CAD build for the part. Positions are in the model's coordinates, mm. A direction names the side the tool comes from. Round coordinates to 2 decimals unless told otherwise and drop trailing zeros. Order: outer loops, then holes, each group sorted by start corner. A loop starts at its lowest first (then second) coordinate and runs counter-clockwise, first axis right, second up. Notation, with made-up numbers: (-17, 89) - (34, 89) arc R27 ccw to (34, 124) - close; hole circle Ø5 at (-17.75, 73). An arc over 180 degrees is marked (long way). Write item = value, one per line.
from build123d import *

# Parameters (mm, degrees)
ESBO_O1_W                = 20
ESBO_O1_H                = 6
RESSALTO_EXTRUS_O1_DEPTH = 40
ESBO_O2_W                = 10
ESBO_O2_H                = 5
ESBO_O2_W_2              = 5
ESBO_O2_H_2              = 10
RESSALTO_EXTRUS_O2_DEPTH = 6
ESBO_O3_R                = 1
CORTE_EXTRUS_O1_DEPTH    = 40
ESBO_O4_R                = 1
CORTE_EXTRUS_O2_DEPTH    = 40
ESBO_O5_R                = 1
CORTE_EXTRUS_O3_DEPTH    = 40
ESBO_O6_R                = 1
CORTE_EXTRUS_O4_DEPTH    = 40
ESBO_O7_W                = 14
ESBO_O7_H                = 13
CORTE_EXTRUS_O5_DEPTH    = 40


with BuildPart() as part:
    # Esboço1 → Ressalto-extrusão1 (new body)
    with BuildSketch(Plane.XY):
        with Locations((0.415187471, 0.908205796)):
            Rectangle(ESBO_O1_W, ESBO_O1_H)
    extrude(amount=RESSALTO_EXTRUS_O1_DEPTH)

    # Esboço2 → Ressalto-extrusão2 (add, through all)
    with BuildSketch(Plane(origin=(0, 3.908205796, 0), x_dir=(1, 0, 0), z_dir=(0, 1, 0))):
        with Locations((-14.584812529, -7.5)):
            Rectangle(ESBO_O2_W, ESBO_O2_H)
        with Locations((-14.584812529, -32.5)):
            Rectangle(ESBO_O2_W, ESBO_O2_H)
        with Locations((-7.084812529, 5)):
            Rectangle(ESBO_O2_W_2, ESBO_O2_H_2)
        with Locations((2.915187471, 5)):
            Rectangle(ESBO_O2_W_2, ESBO_O2_H_2)
        with Locations((15.415187471, -12.5)):
            Rectangle(ESBO_O2_W, ESBO_O2_H)
        with Locations((15.415187471, -27.5)):
            Rectangle(ESBO_O2_W, ESBO_O2_H)
        with Locations((-2.084812529, -45)):
            Rectangle(ESBO_O2_W_2, ESBO_O2_H_2)
        with Locations((7.915187471, -45)):
            Rectangle(ESBO_O2_W_2, ESBO_O2_H_2)
    extrude(amount=-RESSALTO_EXTRUS_O2_DEPTH)

    # Esboço3 → Corte-extrusão1 (cut)
    with BuildSketch(Plane.XY.offset(30)):
        with Locations((16.415187471, 0.908205796)):
            Circle(ESBO_O3_R)
    extrude(amount=-CORTE_EXTRUS_O1_DEPTH, mode=Mode.SUBTRACT)

    # Esboço4 → Corte-extrusão2 (cut)
    with BuildSketch(Plane.ZY.offset(4.584812529)):
        with Locations((46, 0.908205796)):
            Circle(ESBO_O4_R)
    extrude(amount=-CORTE_EXTRUS_O2_DEPTH, mode=Mode.SUBTRACT)

    # Esboço5 → Corte-extrusão3 (cut)
    with BuildSketch(Plane.XY.offset(35)):
        with Locations((-15.584812529, 0.908205796)):
            Circle(ESBO_O5_R)
    extrude(amount=-CORTE_EXTRUS_O3_DEPTH, mode=Mode.SUBTRACT)

    # Esboço6 → Corte-extrusão4 (cut)
    with BuildSketch(Plane(origin=(5.415187471, 0, 0), x_dir=(0, 0, -1), z_dir=(1, 0, 0))):
        with Locations((6, 0.908205796)):
            Circle(ESBO_O6_R)
    extrude(amount=-CORTE_EXTRUS_O4_DEPTH, mode=Mode.SUBTRACT)

    # Esboço7 → Corte-extrusão5 (cut)
    with BuildSketch(Plane(origin=(0, 3.908205796, 0), x_dir=(1, 0, 0), z_dir=(0, 1, 0))):
        with Locations((0.415187471, -9.5)):
            Rectangle(ESBO_O7_W, ESBO_O7_H)
        with Locations((0.415187471, -30.5)):
            Rectangle(ESBO_O7_W, ESBO_O7_H)
    extrude(amount=-CORTE_EXTRUS_O5_DEPTH, mode=Mode.SUBTRACT)


solid = part.part
(1) Pull direction Z, two halves, no side cores. Call faces 5 (the cylindrical face through (-16.584, 0.952, 32.535)), 6 (the flat face through (0, 1, 24)), 7 (the flat face through (15, 1, 30)): released by +Z, released by -Z, zero draft, split by the parting line, or undercut.
Solved:
face_5 = zero draft
face_6 = undercut
face_7 = released by +Z
(2) Band-saw the part on B-B on z = 4. List the corners of the cut face in (x, y).
Solved:
outline = (-9.58, -2.09) - (-6.58, -2.09) - (-6.58, 3.91) - (-9.58, 3.91) - close; (7.42, -2.09) - (10.42, -2.09) - (10.42, 3.91) - (7.42, 3.91) - close
(3) Tool access for faces 1 (the flat face through (-15, 2, 5)), 2 (the flat face through (5.415, 2, 45)), 3 (the flat face through (7.415, 1, 10)), 4 (the flat face through (-7, 1, 40)): list every direction of +Z, -Z, +X, -X, +Y, -Y with a clear straight run to the whole face (end or side of a thin tool).
Solved:
face_1 = -Z, -X, +Y, -Y
face_2 = +Z, +Y, -Y
face_3 = +Y, -Y
face_4 = +Z, -X, +Y, -Y
(4) Band-saw the part on C-C on x = -11. List the corners of the cut face in (y, z).
Solved:
outline = (-2.09, 5) - (3.91, 5) - (3.91, 10) - (-2.09, 10) - close; (-2.09, 30) - (3.91, 30) - (3.91, 35) - (-2.09, 35) - close
(5) Band-saw the part on A-A on z = -6. List the corners of the cut face in (x, y).
Solved:
outline = (-9.58, -2.09) - (-4.58, -2.09) - (-4.58, -0.09) - (-9.58, -0.09) - close; (-9.58, 1.91) - (-4.58, 1.91) - (-4.58, 3.91) - (-9.58, 3.91) - close; (0.42, -2.09) - (5.42, -2.09) - (5.42, -0.09) - (0.42, -0.09) - close; (0.42, 1.91) - (5.42, 1.91) - (5.42, 3.91) - (0.42, 3.91) - close
(6) Probe line 1 along Z through (x, y) = (4, 3.15); line 2 along Z through (x, y) = (13, 2.9); line 3 along X through (y, z) = (0.85, 13). List the from-to ranges inside material, lowest first.
Solved:
line_1 = -10 to 3, 16 to 24, 37 to 40
line_2 = 10 to 15, 25 to 30
line_3 = -9.58 to -6.58, 7.42 to 15.42, 17.41 to 20.42
(7) Band-saw the part on D-D on x = 6.5. List the corners of the cut face in (y, z), plus the area to 3 significant figures.
Solved:
outline = (-2.09, 0) - (3.91, 0) - (3.91, 3) - (-2.09, 3) - close; (-2.09, 16) - (3.91, 16) - (3.91, 24) - (-2.09, 24) - close; (-2.09, 37) - (3.91, 37) - (3.91, 50) - (-2.09, 50) - close; hole circle Ø2 at (0.91, 46)
area = 141 mm²
(8) Drop flat-ended pins along their axis: pin 1 (1.8 mm diameter, centred on x = -13.5, y = -0.5, fed in from -Z); pin 2 (2.5 mm diameter, centred on y = 0.91, z = 46, fed in from +X); pin 3 (1.8 mm diameter, centred on x = 15, y = 1.5, fed in from -Z). Give the stop position or say it passes through.
Solved:
pin_1 = 5
pin_2 = 10.42
pin_3 = 10
